Model file for the job. Use its own axes, mm. Face numbers are marked on the shaded views. Round coordinates to 2 decimals unless told otherwise and drop trailing zeros. Order: outer loops, then holes, each group sorted by start corner. A loop starts at its lowest first (then second) coordinate and runs counter-clockwise, first axis right, second up. Notation, with made-up numbers: (-15.75, -3.5) -> (33.25, -3.5) arc R24 ccw to (33.25, 33.5) -> close; hole circle Ø9 at (70.25, -16.75). An arc over 180 degrees is marked (long way). Answer as CSV lines item,"result".
Autodesk Inventor part; units mm, degrees
ref_plane "Work Plane1" through (-6.4, 0, -14.5) normal (0, -0.9633, -0.2685) x (1, 0, 0)
ref_plane "YZ Plane" through (0, 0, 0) normal (1, 0, 0) x (0, 1, 0)
ref_plane "XZ Plane" through (0, 0, 0) normal (0, 1, 0) x (-1, 0, 0)
sketch "Sketch1" plane through (0, 0, 0) normal (0, 1, 0) x (-1, 0, 0)
  line L0 (0, 0) -> (6.4, 0)
  line L1 (6.4, 0) -> (6.4, -20.6)
  line L2 (6.4, -20.6) -> (0, -20.6)
  line L3 (0, -20.6) -> (0, 0)
  point P0 (3.2, -7.9)
  dimension "d0" = 6.4
  dimension "d1" = 20.6
extrude "Extrusion1" add sketch "Sketch1" along normal blind 3.2
sketch "Sketch3" plane through (0, 0, 0) normal (0, -1, 0) x (1, 0, 0)
  point P0 (0, 0)
  point P1 (-3.2, -5)
hole "Hole1" at (-3.2, 0, -5) direction (0, 1, 0) diameter 4.6 end through all
chamfer "Chamfer1" distance 1.1 angle 45 1 edges at (0, 1.6, 0)
chamfer "Chamfer2" distance 1.1 angle 45 1 edges at (-6.4, 1.6, 0)
chamfer "Chamfer3" distance 1.1 angle 45 1 edges at (-6.4, 1.6, -20.6)
chamfer "Chamfer4" distance 1.1 angle 45 1 edges at (0, 1.6, -20.6)
sketch "Sketch5" plane through (0, 0, 0) normal (1, 0, 0) x (0, 1, 0)
  line L0 (3.2, -20.6) -> (0, -20.6)
  line L1 (0, -20.6) -> (0, -14.5)
  line L2 (0, -1.1) -> (0, -19.5)
  line L3 (0, -20.6) -> (1.7, -20.6)
  line L4 (1.7, -20.6) -> (0, -14.5)
  point P0 (0, 0)
  dimension "d26" = 6.1
  dimension "d27" = 1.7
extrude "Extrusion3" cut sketch "Sketch5" against normal through all
ref_plane "Work Plane1" through (-6.4, 0, -14.5) normal (0, -0.9633, -0.2685) x (1, 0, 0)
sketch "Sketch11" plane through (-6.4, 0, -14.5) normal (0, -0.9633, -0.2685) x (1, 0, 0)
  circle A0 centre (3.2, -2.1) radius 2.01
  line L0 (0, 0) -> (6.4, 0)
  point P0 (6.4, 13.9677)
  dimension "d31" = 4.02
  dimension "d34" = 2.1
extrude "Extrusion4" cut sketch "Sketch11" along normal mid plane 4.2
properties part number "HeadbarClamp"
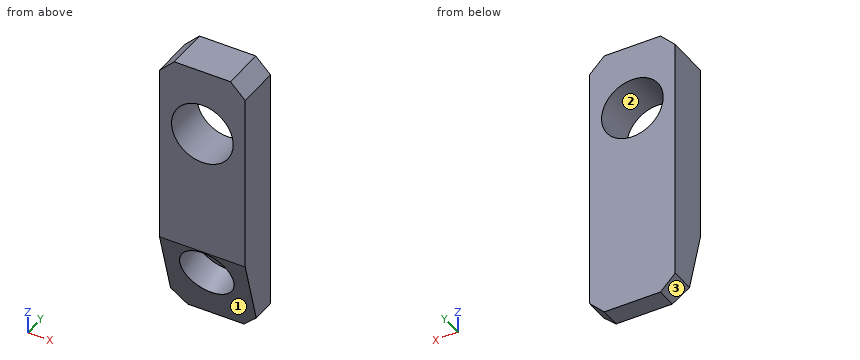
Q1. Wall check: L1, parallel to Z at x = -3.2, y = 1.9; L2, parallel to X at y = 0.7, z = -5; L3, parallel to Z at x = -3.2, y = 0.75. Give the ranges that are in metal, low to high. Write a range as [from, to].
Checks:
L1,"[-20.6, -18.24], [-14.06, -7.3], [-2.7, 0]"
L2,"[-6.4, -5.5], [-0.9, 0]"
L3,"[-14.38, -7.3], [-2.7, 0]"
Q2. Saw through at B-B (x = -3.2). Write the cut outline in (y, z), plus the area to 3 significant figures.
Checks:
outline,"(0, -14.5) -> (0.02, -14.59) -> (2.05, -14.02) -> (3.13, -17.89) -> (1.1, -18.46) -> (1.7, -20.6) -> (3.2, -20.6) -> (3.2, -7.3) -> (0, -7.3) -> close; (0, -2.7) -> (3.2, -2.7) -> (3.2, 0) -> (0, 0) -> close"
area,"37.6 mm²"
Q3. Saw through at A-A (z = -5). Write the cut outline in (x, y), plus the area to 3 significant figures.
Checks:
outline,"(-6.4, 0) -> (-5.5, 0) -> (-5.5, 3.2) -> (-6.4, 3.2) -> close; (-0.9, 0) -> (0, 0) -> (0, 3.2) -> (-0.9, 3.2) -> close"
area,"5.76 mm²"
Q4. Mould opens along X. For the marked faces 1, 2 and 3 say: +X half, -X half, draft (parallel to the pull), parting line (faces both ways), or undercut.
Checks:
face 1,"draft"
face 2,"undercut"
face 3,"-X half"
Q5. Saw through at D-D (x = -2.25). Write the cut outline in (y, z).
Checks:
outline,"(0, -14.5) -> (0.09, -14.82) -> (2.11, -14.25) -> (3.06, -17.66) -> (1.04, -18.23) -> (1.7, -20.6) -> (3.2, -20.6) -> (3.2, -7.09) -> (0, -7.09) -> close; (0, -2.91) -> (3.2, -2.91) -> (3.2, 0) -> (0, 0) -> close"
Q6. Saw through at C-C (x = -6). Write the cut outline in (y, z).
Checks:
outline,"(0, -14.5) -> (1.5, -19.9) -> (3.2, -19.9) -> (3.2, -0.7) -> (0, -0.7) -> close"
